Geometry check sheet. Reference: the model listing, model coordinates, mm. Give positions to 0.01 mm unless a question says otherwise; leave off trailing zeros. Write each loop counter-clockwise with the first axis right and the second up, starting at its lowest first coordinate (ties: lowest second). Pieces come first, ordered by that corner, then holes. Notation, with made-up numbers: M 6.5,-8 L 21.5,-8 A16 ccw 21.5,2 Z; hole C 59,16.5 d1. An arc over 180 degrees is marked long. Write each question's results on one line, items separated by ' | '.
```python
from build123d import *

# Parameters (mm, degrees)
SKETCH1_W             = 51.181
SKETCH1_H             = 44.45
BOSS_EXTRUDE1_DEPTH   = 6.35
BOSS_EXTRUDE2_DEPTH   = 44.45
M4X0_7_TAPPED_HOLE1_D = 3.3


with BuildPart() as part:
    # Sketch1 → Boss-Extrude1 (new body)
    with BuildSketch(Plane(origin=(0, 0, 0), x_dir=(1, 0, 0), z_dir=(0, 1, 0))):
        Rectangle(SKETCH1_W, SKETCH1_H)
    extrude(amount=BOSS_EXTRUDE1_DEPTH)

    # Sketch2 → Boss-Extrude2 (add)
    with BuildSketch(Plane.XY.offset(22.225)):
        with BuildLine():
            Line((-25.5905, 0), (25.5905, 0))
            ThreePointArc((25.5905, 0), (0, -5.696875973), (-25.5905, 0))
        make_face()
    extrude(amount=-BOSS_EXTRUDE2_DEPTH)

    # M4x0.7 Tapped Hole1 (through all)
    with Locations(Plane(origin=(0, 6.35, 0), x_dir=(1, 0, 0), z_dir=(0, 1, 0))):
        with Locations((0, 14.65), (-17.950000041, -14.65), (17.950000041, -14.65)):
            Hole(M4X0_7_TAPPED_HOLE1_D / 2)


solid = part.part
```
Q1. Section check B-B (z = 14.65). State how many separate pieces and enclosed holes the cut face has, then the cut area to 3 significant figures.
Answer key:
separate pieces: 3 | enclosed holes: 0 | area: 460 mm2
Q2. Material ranges on probe 1 along Z at (x, y) = (17.95, 0.75) (3 decimals); probe 2 along X at (y, z) = (-1, 15); probe 3 along Z at (x, y) = (0, -1.5) (3 decimals), recorded low to high. Write a range as [from, to].
Answer key:
probe 1: z = [-22.225, 13], [16.3, 22.225] | probe 2: x = [-23.34, -19.56], [-16.34, 16.34], [19.56, 23.34] | probe 3: z = [-22.225, -16.3], [-13, 22.225]
Q3. Section check A-A (x = 0). Enter the section's corners in (y, z) (3 decimals).
Answer key:
outline: M -5.697,-22.225 L 6.35,-22.225 L 6.35,-16.3 L -5.697,-16.3 Z; M -5.697,-13 L 6.35,-13 L 6.35,22.225 L -5.697,22.225 Z
Q4. Depth check by flat-ended pin: P1, Ø5, axis at x = -10.5, z = -17.5, coming from the -Y side; P2, Ø4.5, axis at x = -17.95, z = 14.65, coming from the -Y side; P3, Ø4, axis at x = 8.5, z = -15, coming from the -Y side. Enter the tip coordinate at first touch or a pass-through.
Answer key:
P1: stops at y = -5.16 | P2: stops at y = -3.62 | P3: stops at y = -5.35
Q5. Section check D-D (y = -4.5). Enter the section's corners in (x, z) (3 decimals), then the cut area to 3 significant figures.
Answer key:
outline: M -11.957,-22.225 L 11.957,-22.225 L 11.957,22.225 L -11.957,22.225 Z; hole C 0,-14.65 d3.3 | area: 1,050 mm2
Q6. Release check for a two-part mould opening along X. For faces 1 (the face through (25.59, 3, 0)), 2 (the face through (-25.59, 3, 0)), 3 (the face through (16.426, 1.38, 15.282)) record: released by +X, released by -X, zero draft, split by the parting line, or undercut.
Answer key:
face 1: released by +X | face 2: released by -X | face 3: undercut
